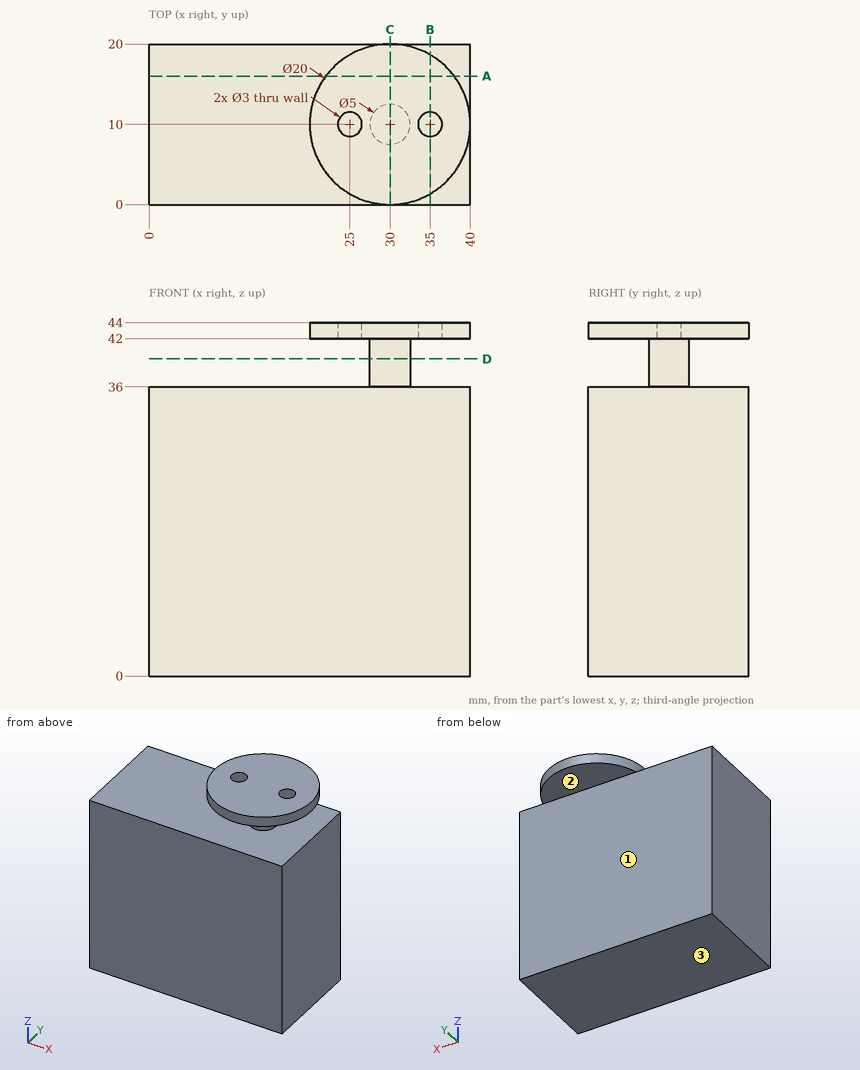
Source: three-view drawing plus pictorial views. Frame: mm from the lowest corner of the part. Coordinates: 2 decimals unless noted, no trailing zeros. Write each loop counter-clockwise with the first axis right and the second up, starting at its lowest first coordinate (ties: lowest second). Pieces come first, ordered by that corner, then holes. Notation, with made-up numbers: (79, 9) -> (95, 9) arc R25 cw to (95, 45) -> close; hole circle Ø3 at (13, 26.5). An arc over 180 degrees is marked (long way). Answer as a JSON object with one key per item and string values.
1. Section D-D on z = 39.5. Return the cut outline in (x, y), then the cut area to 3 significant figures.
Result set:
{"outline": "circle Ø5 at (30, 10)", "area": "19.6 mm2"}
2. Section C-C on x = 30. Return the cut outline in (y, z).
Result set:
{"outline": "(0, 0) -> (20, 0) -> (20, 36) -> (12.5, 36) -> (12.5, 42) -> (20, 42) -> (20, 44) -> (0, 44) -> (0, 42) -> (7.5, 42) -> (7.5, 36) -> (0, 36) -> close"}
3. Section A-A on y = 16. Return the cut outline in (x, z), then the cut area to 3 significant figures.
Result set:
{"outline": "(0, 0) -> (40, 0) -> (40, 36) -> (0, 36) -> close; (22, 42) -> (38, 42) -> (38, 44) -> (22, 44) -> close", "area": "1,470 mm2"}
4. Material intervals for line 1 (Z direction, x = 21.5, y = 12.25); line 2 (Z direction, x = 17, y = 17.25); line 3 (Y direction, x = 25, z = 43.1), sorted ascending. Write a range as from..to.
Result set:
{"line 1": "z = 0..36, 42..44", "line 2": "z = 0..36", "line 3": "y = 1.34..8.5, 11.5..18.66"}
5. Section B-B on x = 35. Return the cut outline in (y, z), then the cut area to 3 significant figures.
Result set:
{"outline": "(0, 0) -> (20, 0) -> (20, 36) -> (0, 36) -> close; (1.34, 42) -> (8.5, 42) -> (8.5, 44) -> (1.34, 44) -> close; (11.5, 42) -> (18.66, 42) -> (18.66, 44) -> (11.5, 44) -> close", "area": "749 mm2"}
6. Mould query, pull axis Z, two halves, no side actions, for the marked faces 1, 2 and 3. Classes: released by +Z, released by -Z, zero draft, split by the parting line, or undercut.
Result set:
{"face 1": "zero draft", "face 2": "undercut", "face 3": "released by -Z"}
